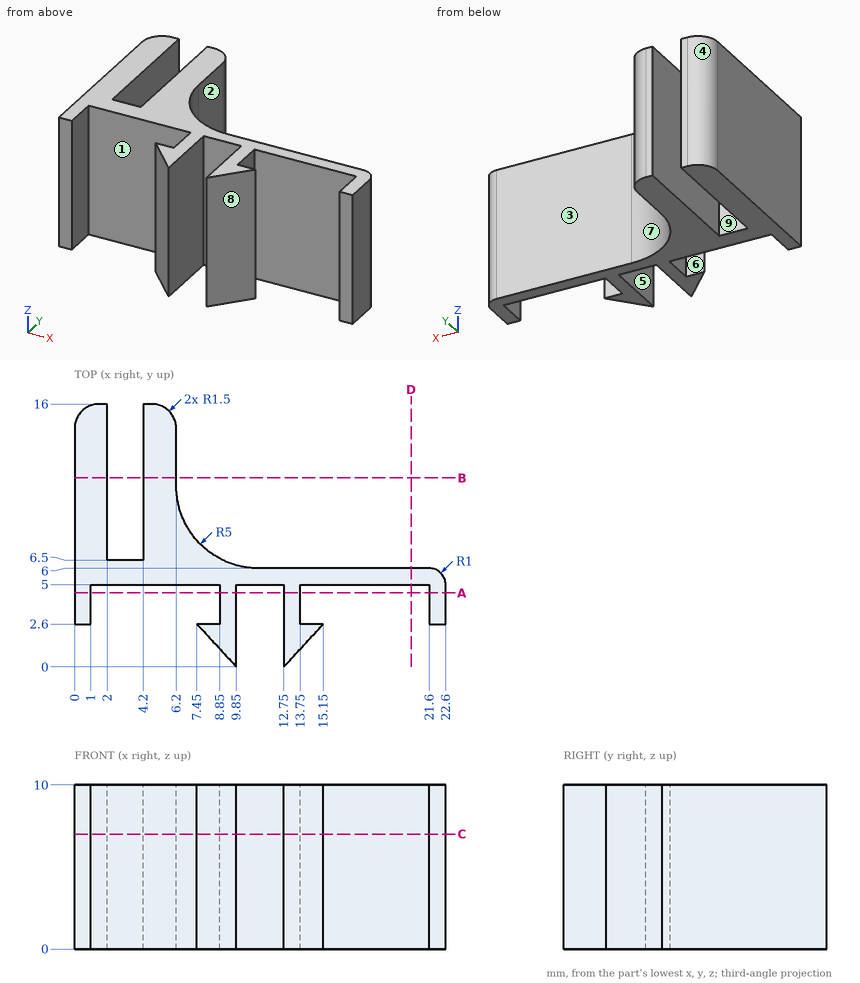
For this review, use the dimensioned drawing (mm, ordinates from the lowest corner) and the shaded views. A direction names the side the tool comes from. Give positions to 0.01 mm unless a question says otherwise; leave off trailing zeros. Write each loop counter-clockwise with the first axis right and the second up, starting at its lowest first coordinate (ties: lowest second). Pieces come first, ordered by that corner, then holes. Notation, with made-up numbers: M 27,-31.5 L 86,-31.5 A25 ccw 86,-5.5 Z; hole C -5,17.25 d2. An arc over 180 degrees is marked long. Answer as a JSON object with one key per item and string values. Group by question number.
Item 1: Tool access review of the marked faces 5, 6, 7, 8 and 9: name each direction out of +Z, -Z, +X, -X, +Y, -Y from which nothing blocks a thin tool from reaching the whole face with its end or side.
Item 2: Consider section B-B on y = 11.5. Write out the cut boundary in (x, z).
Item 3: Consider section D-D on x = 20.5. Write out the cut boundary in (y, z).
Item 4: For probe 1 along X at (y, z) = (4.5, 8.25); probe 2 along X at (y, z) = (13.25, 6.5); probe 3 along Y at (x, z) = (12.25, 8.5), list the stretches that pass through material, from the lowest coordinate up. Write a range as [from, to].
Item 5: Consider section C-C on z = 7. Write out the cut boundary in (x, y), plus the area to 3 significant figures.
Item 6: Draft analysis for pull direction X (two halves, no side actions). For the marked faces 1, 2, 3 and 4, state which applies: +X half, -X half, draft (parallel to the pull), parting line (faces both ways), or undercut.
Item 7: For pin 1 Ø1.9 at (y, z) = (4, 6) entering from -X; pin 2 Ø1.1 at (x, z) = (8, 3.5) entering from +Y; pin 3 Ø1.1 at (x, z) = (14.5, 2.5) entering from +Y; pin 4 Ø2 at (x, z) = (8, 1) entering from +Y, all flat-tipped, find the tip position at first contact; note any pin that passes through.
Item 8: Consider section A-A on y = 4.5. Write out the cut boundary in (x, z), plus the area to 3 significant figures.
Check result:
{
 "1": {"face 5": "+Z, -Z, -Y", "face 6": "+Z, -Z", "face 7": "+Z, -Z, +X, +Y", "face 8": "+Z, -Z, +X, -Y", "face 9": "+Z, -Z, +Y"},
 "2": {"outline": "M 0,0 L 2,0 L 2,10 L 0,10 Z; M 4.2,0 L 6.2,0 L 6.2,10 L 4.2,10 Z"},
 "3": {"outline": "M 5,0 L 6,0 L 6,10 L 5,10 Z"},
 "4": {"probe 1": "x = [0, 1], [8.85, 9.85], [12.75, 13.75], [21.6, 22.6]", "probe 2": "x = [0, 2], [4.2, 6.2]", "probe 3": "y = [5, 6]"},
 "5": {"outline": "M 0,2.6 L 1,2.6 L 1,5 L 8.85,5 L 8.85,2.6 L 7.45,2.6 L 9.85,0 L 9.85,5 L 12.75,5 L 12.75,0 L 15.15,2.6 L 13.75,2.6 L 13.75,5 L 21.6,5 L 21.6,2.6 L 22.6,2.6 L 22.6,5 A1 ccw 21.6,6 L 11.2,6 A5 cw 6.2,11 L 6.2,14.5 A1.5 ccw 4.7,16 L 4.2,16 L 4.2,6.5 L 2,6.5 L 2,16 L 1.5,16 A1.5 ccw 0,14.5 Z", "area": "83.7 mm^2"},
 "6": {"face 1": "undercut", "face 2": "+X half", "face 3": "draft", "face 4": "-X half"},
 "7": {"pin 1": "stops at x = 0", "pin 2": "stops at y = 7.69", "pin 3": "stops at y = 6", "pin 4": "stops at y = 8.29"},
 "8": {"outline": "M 0,0 L 1,0 L 1,10 L 0,10 Z; M 8.85,0 L 9.85,0 L 9.85,10 L 8.85,10 Z; M 12.75,0 L 13.75,0 L 13.75,10 L 12.75,10 Z; M 21.6,0 L 22.6,0 L 22.6,10 L 21.6,10 Z", "area": "40.0 mm^2"}
}
